```python
from build123d import *

# Parameters (mm, degrees)
SKETCH4_R           = 8.5
SKETCH4_W           = 20
SKETCH4_H           = 3
BOSS_EXTRUDE2_DEPTH = 3


with BuildPart() as part:
    # Sketch4 → Boss-Extrude2 (new body)
    with BuildSketch(Plane.XY):
        Polygon((62, 90), (-30, 52.5), (-30, 22.5), (-62, 22.5), (-62, 10), (-65, 10), (-65, -10), (-62, -10), (-62, -22.5), (-10, -22.5), (-10, -25.5), (10, -25.5), (10, -22.5), (62, -22.5), (62, -10), (65, -10), (65, 10), (62, 10), (62, 22.5), (62, 30), (65, 30), (65, 50), (62, 50), (62, 70), (65, 70), (65, 90), align=None)
        with Locations((-12, -7.5)):
            Circle(SKETCH4_R, mode=Mode.SUBTRACT)
        with Locations((12, -7.5)):
            Circle(SKETCH4_R, mode=Mode.SUBTRACT)
        with BuildLine():
            Line((-3.5, -13.5), (3.5, -13.5))
            ThreePointArc((3.5, -13.5), (6, -16), (3.5, -18.5))
            Line((3.5, -18.5), (-3.5, -18.5))
            ThreePointArc((-3.5, -18.5), (-6, -16), (-3.5, -13.5))
        make_face(mode=Mode.SUBTRACT)
        with BuildLine():
            Line((4, -1.5), (-4, -1.5))
            ThreePointArc((-4, -1.5), (-5.414213562, -0.914213562), (-6, 0.5))
            Line((-6, 0.5), (-6, 1.5))
            Line((-6, 1.5), (6, 1.5))
            Line((6, 1.5), (6, 0.5))
            ThreePointArc((6, 0.5), (5.414213562, -0.914213562), (4, -1.5))
        make_face(mode=Mode.SUBTRACT)
        with Locations((0, 24)):
            Rectangle(SKETCH4_W, SKETCH4_H, mode=Mode.SUBTRACT)
        with Locations((40, 24)):
            Rectangle(SKETCH4_W, SKETCH4_H, mode=Mode.SUBTRACT)
    extrude(amount=BOSS_EXTRUDE2_DEPTH)


solid = part.part
```
Model file for the job. Use its own axes, mm. A direction names the side the tool comes from. Give positions to 0.01 mm unless a question says otherwise; leave off trailing zeros. Loops run counter-clockwise (first coordinate to the right, second up) from the corner with the lowest first, then second, coordinate; pieces in that order, holes last. Notation, with made-up numbers: (58.25, 43.5) -> (94.25, 43.5) arc R28 cw to (94.25, 73.5) -> close; hole circle Ø2 at (25, 29.25). An arc over 180 degrees is marked (long way). Use CSV: the item, a comma, the result in double quotes. Start each with the question number.
1) Slice it at A-A on x = 13.5. Give the cut face in (y, z).
2) Slice it at D-D on x = -12. Give the cut face in (y, z), plus the area to 3 significant figures.
3) Wall check: line 1 (X direction, y = -11.5, z = 2.55); line 2 (Y direction, x = -38.5, z = 2.4); line 3 (Y direction, x = 12, z = 1.9). Give the ranges that are in metal, low to high.
4) Slice it at B-B on z = 2.05. Give the number of separate pieces and of enclosed holes in the cut face, plus the area to 3 significant figures.
5) Mould opens along X. For faces 5 (the flat face through (65, 80, 1)), 6 (the flat face through (64, 90, 1)), 7 (the flat face through (0, 25.5, 1)) say: released by +X, released by -X, zero draft, split by the parting line, or undercut.
6) Tool access for faces 1 (the flat face through (-30, 38, 1)), 2 (the flat face through (62, -16, 1)), 3 (the flat face through (0, -18.5, 1)), 4 (the flat face through (-10, -24, 1)): list every direction of +Z, -Z, +X, -X, +Y, -Y with a clear straight run to the whole face (end or side of a thin tool).
7) Flat gauge pins, fed straight in: pin 1 Ø1 at (x, z) = (15.5, 1) entering from +Y; pin 2 Ø1.5 at (y, z) = (17.5, 2) entering from -X; pin 3 Ø1.5 at (y, z) = (23.5, 2) entering from +X. Where does each tip first touch, or does it go through?
8) Slice it at C-C on y = 34.5. Give the cut face in (x, z), plus the area to 3 significant figures.
Computed values:
1,outline,"(-22.5, 0) -> (-15.87, 0) -> (-15.87, 3) -> (-22.5, 3) -> close; (0.87, 0) -> (70.23, 0) -> (70.23, 3) -> (0.87, 3) -> close"
2,outline,"(-22.5, 0) -> (-16, 0) -> (-16, 3) -> (-22.5, 3) -> close; (1, 0) -> (59.84, 0) -> (59.84, 3) -> (1, 3) -> close"
2,area,"196 mm^2"
3,line 1,"x = -62 to -19.5, -4.5 to 4.5, 19.5 to 62"
3,line 2,"y = -22.5 to 22.5"
3,line 3,"y = -22.5 to -16, 1 to 69.62"
4,separate pieces,"1"
4,enclosed holes,"6"
4,area,"9,700 mm^2"
5,face 5,"released by +X"
5,face 6,"zero draft"
5,face 7,"undercut"
6,face 1,"+Z, -Z, -X, +Y"
6,face 2,"+Z, -Z, +X, -Y"
6,face 3,"+Z, -Z"
6,face 4,"+Z, -Z, -X, -Y"
7,pin 1,"stops at y = 71.25"
7,pin 2,"stops at x = -62"
7,pin 3,"stops at x = 62"
8,outline,"(-30, 0) -> (65, 0) -> (65, 3) -> (-30, 3) -> close"
8,area,"285 mm^2"
